Answer from the drawing. Dimensions are ordinates in mm from the lowest x, y and z of the part. A direction names the side the tool comes from. Round coordinates to 2 decimals unless told otherwise and drop trailing zeros. Loops run counter-clockwise (first coordinate to the right, second up) from the corner with the lowest first, then second, coordinate; pieces in that order, holes last. Notation, with made-up numbers: M -40,56 L -24,56 A29 ccw -24,88 Z; hole C 26.5,-3 d2. An arc over 180 degrees is marked long. One line per item, written item: value.
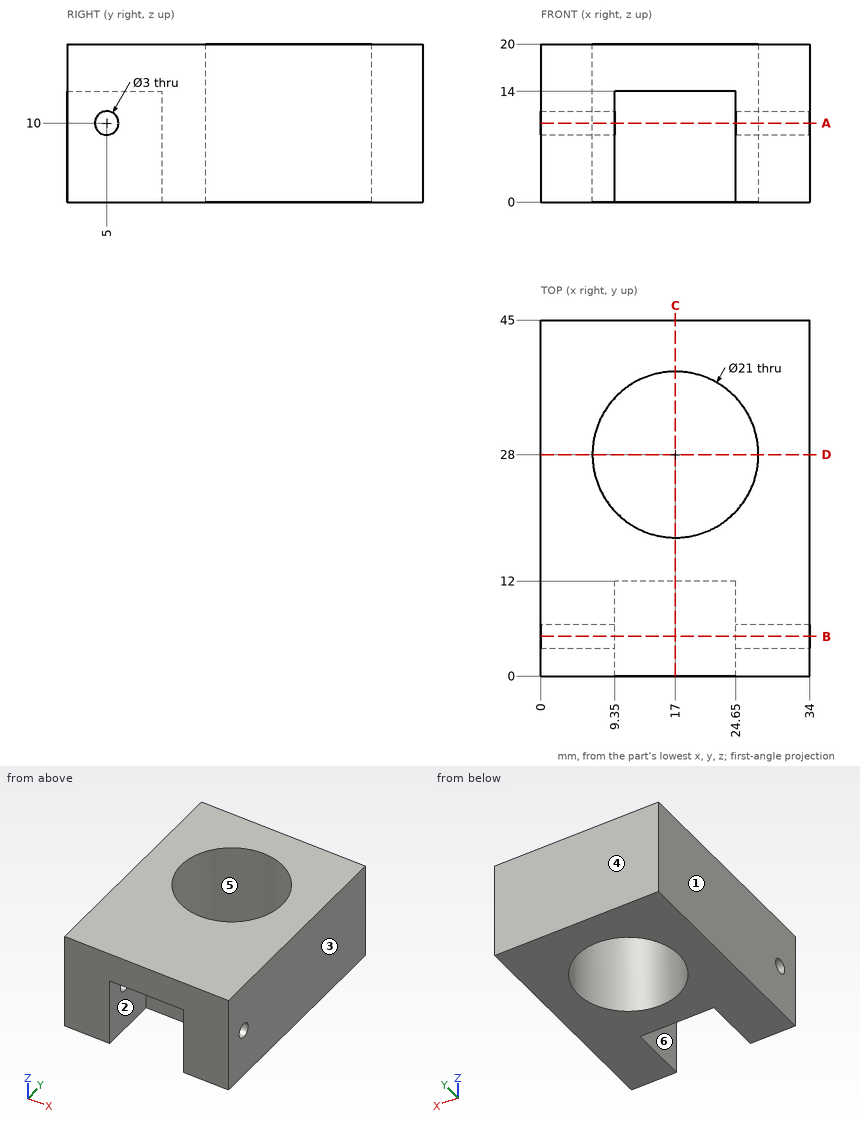
1) Find section D-D (y = 28). Give the vertices of the cut face in (x, z), then the cut area to 3 significant figures.
Check values:
outline: M 0,0 L 6.5,0 L 6.5,20 L 0,20 Z; M 27.5,0 L 34,0 L 34,20 L 27.5,20 Z
area: 260 mm2
2) Find section C-C (x = 17). Give the vertices of the cut face in (y, z).
Check values:
outline: M 0,14 L 12,14 L 12,0 L 17.5,0 L 17.5,20 L 0,20 Z; M 38.5,0 L 45,0 L 45,20 L 38.5,20 Z
3) Find section B-B (y = 5). Give the vertices of the cut face in (x, z).
Check values:
outline: M 0,0 L 9.35,0 L 9.35,8.5 L 0,8.5 Z; M 0,11.5 L 9.35,11.5 L 9.35,14 L 24.65,14 L 24.65,11.5 L 34,11.5 L 34,20 L 0,20 Z; M 24.65,0 L 34,0 L 34,8.5 L 24.65,8.5 Z
4) Find the intervals of material crossed by probe 1 along X at (y, z) = (6, 5.5); probe 2 along Z at (x, y) = (30.25, 5); probe 3 along Y at (x, z) = (14, 12), in increasing order. Write a range as from..to.
Check values:
probe 1: 0..9.35, 24.65..34
probe 2: 0..8.5, 11.5..20
probe 3: 12..17.94, 38.06..45
5) The mould has two halves that part along X. Classify the marked faces 3, 4, 5 and 6: +X half, -X half, draft (parallel to the pull), parting line (faces both ways), or undercut.
Check values:
face 3: +X half
face 4: draft
face 5: undercut
face 6: undercut
6) For the marked faces 1 and 2, determine the directions among +Z, -Z, +X, -X, +Y, -Y from which every point of the face is accessible in a straight line to the end or side of a thin tool.
Check values:
face 1: +Z, -Z, -X, +Y, -Y
face 2: -Z, -Y
7) Find section A-A (z = 10). Give the vertices of the cut face in (x, y).
Check values:
outline: M 0,0 L 9.35,0 L 9.35,3.5 L 0,3.5 Z; M 0,6.5 L 9.35,6.5 L 9.35,12 L 24.65,12 L 24.65,6.5 L 34,6.5 L 34,45 L 0,45 Z; M 24.65,0 L 34,0 L 34,3.5 L 24.65,3.5 Z; hole C 17,28 d21
8) Each of these flat-tipped pins is pushed along its axis until it touches: pin 1 (9.5 mm diameter, centred on x = 13.5, y = 4, fed in from -Z); pin 2 (4 mm diameter, centred on x = 14, z = 6, fed in from -Y). Where does it stop, or does it pass through?
Check values:
pin 1: z = 0
pin 2: y = 12
